Here's how the part is built. I have some questions about the finished solid (model axes, mm). A direction names the side the tool comes from. Round coordinates to 2 decimals unless told otherwise and drop trailing zeros. Write each loop counter-clockwise with the first axis right and the second up, starting at its lowest first coordinate (ties: lowest second). Pieces come first, ordered by that corner, then holes. Notation, with made-up numbers: M -31.75,-20 L -24.75,-20 A30 ccw -24.75,14 Z; hole C 7.25,-26.5 d9. An arc over 180 degrees is marked long. Use one line per item in the form item = value. Start each with the question number.
Q1. I want a section at C-C on y = -15. List the corners of the cut face in (x, z) for me.
Q2. I need wall thicknesses on line 1 along Y through (x, z) = (24.5, 0.8); line 2 along Y through (x, z) = (14.5, 13.65); line 3 along Y through (x, z) = (-14, 5.75). Which ranges of each line are inside material? Lowest first, please. Write a range as from..to.
Q3. I want a section at D-D on z = -0.75. List the corners of the cut face in (x, y) for me.
Q4. For faces 4 (the face through (-25, -4, -5)), 5 (the face through (23, -4, 5.75)), 6 (the face through (-11.5, -3, 4)), 7 (the face through (-10, 6, 7)), which set-ups out of +Z, -Z, +X, -X, +Y, -Y let a thin tool reach every point of the face, with its end or its side?
Q5. We'd pull the mould along X, two halves only. Please class faces 1 (the face through (-6, 15, 5)), 2 (the face through (-26.5, -4, 0)), 3 (the face through (-22, -13, -2)): +X half, -X half, draft (parallel to the pull), parting line (faces both ways), or undercut.
Q6. I want a section at B-B on x = 1. List the corners of the cut face in (y, z) for me.
Q7. I want a section at A-A on z = 9. List the corners of the cut face in (x, y) for me.
Q8. I'm going to push flat-ended pins straight in: pin 1 Ø12 at (x, y) = (-4.5, 4.5) entering from +Z; pin 2 Ø3.5 at (x, y) = (22.5, 5) entering from +Z; pin 3 Ø4 at (x, z) = (-21, 5) entering from +Y; pin 4 Ø5 at (x, z) = (6.5, -4) entering from -Y. Where does each tip first touch, or does it pass through?
Autodesk Inventor part; units mm, degrees
ref_plane "YZ Plane" through (0, 0, 0) normal (1, 0, 0) x (0, 1, 0)
ref_plane "XZ Plane" through (0, 0, 0) normal (0, 1, 0) x (-1, 0, 0)
ref_plane "XY Plane" through (0, 0, 0) normal (0, 0, 1) x (1, 0, 0)
sketch "Base" plane through (0, 0, 0) normal (0, 0, 1) x (1, 0, 0)
  line L0 (26.5, -20) -> (-26.5, -20)
  line L1 (-26.5, -20) -> (-26.5, 20)
  line L2 (-26.5, 20) -> (26.5, 20)
  line L3 (26.5, 20) -> (26.5, -20)
  line L4 (26.5, -20) -> (-26.5, 20) construction
  line L5 (-26.5, -20) -> (26.5, 20) construction
  point P0 (0, 0)
  dimension "d0" = 53
  dimension "d1" = 40
extrude "BaseFeature" add sketch "Base" along normal blind 1.25
fillet "BaseFilletFeature" radius 2 4 edges at (-26.5, 20, 0.625) (26.5, 20, 0.625) (-26.5, -20, 0.625) (26.5, -20, 0.625)
sketch "MountHoles" plane through (0, 0, 1.25) normal (0, 0, 1) x (1, 0, 0)
  arc A0 (-24.5, 20) -> (-26.5, 18) centre (-24.5, 18) ccw
  arc A1 (26.5, 18) -> (24.5, 20) centre (24.5, 18) ccw
  arc A2 (-26.5, -18) -> (-24.5, -20) centre (-24.5, -18) ccw
  arc A3 (24.5, -20) -> (26.5, -18) centre (24.5, -18) ccw
  circle A4 centre (-24.5, 18) radius 1.25
  circle A5 centre (24.5, 18) radius 1.25
  circle A6 centre (-24.5, -18) radius 1.25
  circle A7 centre (24.5, -18) radius 1.25
  point P0 (0, 0)
  dimension "d5" = 2.5
extrude "MountHolesFeature" cut sketch "MountHoles" against normal through all
sketch "Sketch3" plane through (0, 0, 1.25) normal (0, 0, 1) x (1, 0, 0)
  line L0 (26.5, 10) -> (18.5, 10)
  line L1 (18.5, 10) -> (18.5, 2)
  line L2 (18.5, 2) -> (26.5, 2)
  line L3 (26.5, 2) -> (26.5, 10)
  line L4 (26.5, -2) -> (18.5, -2)
  line L5 (18.5, -2) -> (18.5, -10)
  line L6 (18.5, -10) -> (26.5, -10)
  line L7 (26.5, -10) -> (26.5, -2)
  line L8 (24.5, 20) -> (-24.5, 20)
  line L9 (-24.5, -20) -> (24.5, -20)
  line L10 (26.5, -18) -> (26.5, 18)
  point P0 (0, 0)
  point P1 (22.5, 10)
  dimension "d8" = 10
  dimension "d9" = 8
  dimension "d10" = 10
  dimension "d11" = 8
extrude "Extrusion3" add sketch "Sketch3" along normal blind 8.5
sketch "Sketch4" plane through (18.5, -10, 1.25) normal (0, -1, 0) x (1, 0, 0)
  line L0 (0, 0) -> (0, 8.5)
  line L1 (0, 4.25) -> (8, 4.25)
  line L2 (8, 0) -> (8, 8.5)
  line L3 (0, 4.25) -> (1.8922, 8.5)
  line L4 (0, 8.5) -> (8, 8.5)
  line L5 (8, 4.25) -> (6.1078, 8.5)
  point P0 (-18.5, -1.25)
  dimension "d14" = 24
  dimension "d15" = 24
extrude "Extrusion4" cut sketch "Sketch4" along normal through all both and the other way through all contours L0 L4 L3 | L5 L4 L2
sketch "Sketch5" plane through (0, 0, 9.75) normal (0, 0, 1) x (1, 0, 0)
  line L0 (20.3922, 10) -> (20.3922, 2) construction
  line L1 (20.3922, 6) -> (24.6078, 6) construction
  line L2 (24.6078, 2) -> (24.6078, 10) construction
  circle A0 centre (22.5, 7.8922) radius 2.1078 construction
  line L3 (24.6078, 10) -> (20.3922, 10) construction
  circle A1 centre (22.5, 4.1078) radius 2.1078 construction
  line L4 (20.3922, 2) -> (24.6078, 2) construction
  circle A2 centre (22.5, 7.8922) radius 1.5
  circle A3 centre (22.5, 4.1078) radius 1.5
  point P0 (0, 0)
  dimension "d18" = 3
  dimension "d19" = 3
extrude "Extrusion5" cut sketch "Sketch5" against normal blind 4
mirror "Mirror1" about plane through (0, 0, 0) normal (0, 1, 0) of "Extrusion5"
sketch "Sketch6" plane through (0, 0, 1.25) normal (0, 0, 1) x (1, 0, 0)
  circle A0 centre (14.5, 16) radius 4
  line L0 (24.5, 20) -> (-24.5, 20)
  line L1 (10.5, 20) -> (18.5, 20)
  line L2 (18.5, 20) -> (18.5, 12) construction
  line L3 (18.5, 12) -> (10.5, 12) construction
  line L4 (10.5, 12) -> (10.5, 20) construction
  line L5 (26.5, 10) -> (26.5, 18)
  point P0 (0, 0)
  dimension "d22" = 8
  dimension "d23" = 8
extrude "Extrusion6" add sketch "Sketch6" along normal blind 12.5
sketch "Sketch7" plane through (14.5, 16, 13.75) normal (0, 0, 1) x (1, 0, 0)
  circle A0 centre (0, 0) radius 4
  circle A1 centre (0, 0) radius 3.3
  point P0 (-14.5, -16)
  dimension "d26" = 0.7
extrude "Extrusion7" cut sketch "Sketch7" against normal blind 0.5 contours A1
sketch "Sketch8" plane through (0, 0, 1.25) normal (0, 0, 1) x (1, 0, 0)
  line L0 (-26.5, 18) -> (-26.5, -18)
  line L1 (-26.5, -0.5) -> (-11.5, -0.5)
  line L2 (-11.5, -0.5) -> (-11.5, -6.5)
  line L3 (-11.5, -6.5) -> (-26.5, -6.5)
  line L4 (-26.5, -6.5) -> (-26.5, -0.5)
  line L5 (-24.5, -20) -> (24.5, -20)
  point P0 (0, 0)
  dimension "d29" = 15
  dimension "d30" = 6
  dimension "d31" = 13.5
extrude "Extrusion8" add sketch "Sketch8" along normal blind 5
sketch "Sketch9" plane through (-26.5, -18, 0) normal (-1, 0, 0) x (0, 0, 1)
  line L0 (1.25, 17.5) -> (6.25, 17.5) construction
  line L1 (6.25, 17.5) -> (6.25, 11.5) construction
  line L2 (1.25, 11.5) -> (6.25, 11.5) construction
  circle A0 centre (3.25, 14.5) radius 3 construction
  circle A1 centre (3.25, 14.5) radius 2.5
  circle A2 centre (3.25, 14.5) radius 2
  point P0 (0, 18)
  dimension "d34" = 0.5
  dimension "d35" = 0.5
extrude "Extrusion9" add sketch "Sketch9" along normal blind 2.5
sketch "Sketch10" plane through (0, 0, 1.25) normal (0, 0, 1) x (1, 0, 0)
  line L0 (14.5, 20) -> (-24.5, 20)
  line L1 (-15, 20) -> (-6, 20)
  line L2 (-6, 20) -> (-6, 6)
  line L3 (-6, 6) -> (-15, 6)
  line L4 (-15, 6) -> (-15, 20)
  line L5 (-26.5, 18) -> (-26.5, -0.5)
  point P0 (0, 0)
  dimension "d38" = 14
  dimension "d39" = 9
  dimension "d40" = 11.5
extrude "Extrusion10" add sketch "Sketch10" along normal blind 11
sketch "Sketch11" plane through (-24.5, 20, 0) normal (0, 1, 0) x (1, 0, 0)
  line L0 (18.5, -1.25) -> (18.5, -12.25) construction
  line L1 (18.5, -12.25) -> (9.5, -12.25) construction
  line L2 (9.5, -1.25) -> (9.5, -12.25) construction
  circle A0 centre (14, -7.75) radius 4.5
  circle A1 centre (14, -7.75) radius 4
  circle A2 centre (14, -7.75) radius 0.125
  point P0 (24.5, 0)
  dimension "d43" = 0.5
  dimension "d44" = 0.25
extrude "Extrusion11" cut sketch "Sketch11" against normal blind 11 contours A1
sketch "Sketch12" plane through (0, 0, 1.25) normal (0, 0, 1) x (1, 0, 0)
  line L0 (-4.5, -4.5) -> (4.5, -4.5)
  line L1 (4.5, -4.5) -> (4.5, 4.5)
  line L2 (4.5, 4.5) -> (-4.5, 4.5)
  line L3 (-4.5, 4.5) -> (-4.5, -4.5)
  line L4 (-4.5, -4.5) -> (4.5, 4.5) construction
  line L5 (4.5, -4.5) -> (-4.5, 4.5) construction
  point P0 (0, 0)
  dimension "d47" = 9
extrude "Extrusion12" add sketch "Sketch12" along normal blind 0.5
sketch "Sketch13" plane through (-15, 6, 1.25) normal (0, -1, 0) x (1, 0, 0)
  circle A0 centre (4.5, 6.5) radius 4
  circle A1 centre (4.5, 6.5) radius 4.5
  line L0 (9, 0) -> (0, 0)
  line L1 (9, 0) -> (9, 11)
  line L2 (0, 11) -> (9, 11)
  line L3 (0, 0) -> (0, 11)
  point P0 (15, -1.25)
  point P1 (0, 6.5)
  point P2 (4.5, 11)
  point P3 (9, 6.5)
extrude "Extrusion13" cut sketch "Sketch13" against normal blind 11.5 contours A1 L2 L1 | A1 L3 L2
sketch "Sketch14" plane through (0, 0, 1.25) normal (0, 0, 1) x (1, 0, 0)
  line L0 (14.5, 20) -> (-6, 20)
  line L1 (10.5, 20) -> (4, 20)
  line L2 (4, 20) -> (4, 10.5)
  line L3 (4, 10.5) -> (10.5, 10.5)
  line L4 (10.5, 10.5) -> (10.5, 20)
  circle A0 centre (14.5, 16) radius 4
  point P0 (0, 0)
  point P1 (4, 20)
  dimension "d52" = 6.5
  dimension "d53" = 9.5
extrude "Extrusion14" add sketch "Sketch14" along normal blind 1 contours L4 L3 L2 L0
sketch "Sketch15" plane through (0, 0, 0) normal (0, 0, -1) x (-1, 0, 0)
  line L0 (26.5, -6.5) -> (26.5, -18)
  line L1 (26.5, -3.5) -> (17, -3.5)
  line L2 (17, -3.5) -> (17, -13)
  line L3 (17, -13) -> (26.5, -13)
  line L4 (26.5, -13) -> (26.5, -3.5)
  line L5 (24.5, -20) -> (-24.5, -20)
  point P0 (0, 0)
  dimension "d56" = 9.5
  dimension "d57" = 7
extrude "Extrusion15" add sketch "Sketch15" along normal blind 5
sketch "Sketch16" plane through (0, 0, -5) normal (0, 0, -1) x (-1, 0, 0)
  line L0 (17, -13) -> (26.5, -13)
  line L1 (26.5, -13) -> (26.5, -3.5)
  line L2 (26.5, -3.5) -> (17, -3.5)
  line L3 (17, -3.5) -> (17, -13)
  circle A0 centre (21.75, -8.25) radius 4.75
  point P0 (0, 0)
extrude "Extrusion16" add sketch "Sketch16" along normal blind 6 draft -2 contours A0
properties part number "Max9744_20W_ClassD_Amplifier"
Reported:
q1.outline = M -26.5,0 L 26.5,0 L 26.5,1.25 L -26.5,1.25 Z
q2.line_1 = -20..-19.25, -16.75..16.75, 19.25..20
q2.line_2 = 12..12.7, 19.3..20
q2.line_3 = -6.5..-0.5, 6..20
q3.outline = M -26.5,-13 L -17,-13 L -17,-3.5 L -26.5,-3.5 Z
q4.face_4 = -Z, -X, +Y
q4.face_5 = +Z
q4.face_6 = +Z, -Y
q4.face_7 = +Z, -X
q5.face_1 = undercut
q5.face_2 = -X half
q5.face_3 = draft
q6.outline = M -20,0 L 20,0 L 20,1.25 L 4.5,1.25 L 4.5,1.75 L -4.5,1.75 L -4.5,1.25 L -20,1.25 Z
q7.outline = M -15,17.5 L -14.82,17.5 L -14.82,6 L -6.18,6 L -6.18,17.5 L -6,17.5 L -6,20 L -6.7,20 L -6.7,9 L -14.3,9 L -14.3,20 L -15,20 Z; C 14.5,16 d8; M 20.06,-10 L 24.94,-10 L 24.94,-2 L 20.06,-2 Z; M 20.06,2 L 24.94,2 L 24.94,10 L 20.06,10 Z; hole C 22.5,-7.89 d3; hole C 22.5,-4.11 d3; hole C 22.5,4.11 d3; hole C 22.5,7.89 d3
q8.pin_1 = 12.25
q8.pin_2 = 9.75
q8.pin_3 = -0.5
q8.pin_4 = through
